Model file for the job. Use its own axes, mm. Face numbers are marked on the shaded views. Round coordinates to 2 decimals unless told otherwise and drop trailing zeros. Loops run counter-clockwise (first coordinate to the right, second up) from the corner with the lowest first, then second, coordinate; pieces in that order, holes last. Notation, with made-up numbers: (-11, -37.5) -> (17, -37.5) arc R24 cw to (17, -26.5) -> close; hole circle Ø4 at (-29.5, 39.25). An arc over 180 degrees is marked (long way). Use a Markdown table: item, result.
from build123d import *

# Parameters (mm, degrees)
SKETCH_1_W         = 40
SKETCH_1_H         = 40
EXTRUDE_1_DEPTH    = 4
HOLE_WIZARD_M101_D = 11
FILLET_1_R         = 3
HOLE_WIZARD_M61_D  = 6.6


with BuildPart() as part:
    # Эскиз1 → Бобышка-Вытянуть1 (new body)
    with BuildSketch(Plane(origin=(0, 0, 0), x_dir=(1, 0, 0), z_dir=(0, 1, 0))):
        Rectangle(SKETCH_1_W, SKETCH_1_H)
    extrude(amount=EXTRUDE_1_DEPTH)

    # Отверстие с зазором M101 (through all)
    with Locations(Plane(origin=(0, 4, 0), x_dir=(1, 0, 0), z_dir=(0, 1, 0))):
        with Locations((0, 0)):
            Hole(HOLE_WIZARD_M101_D / 2)

    # Скругление1
    fillet_1_edges = [part.edges().sort_by_distance(p)[0] for p in [
        (20, 2, 20),
        (-20, 2, 20),
        (-20, 2, -20),
        (20, 2, -20),
    ]]
    fillet(fillet_1_edges, radius=FILLET_1_R)

    # Отверстие с зазором M61 (through all)
    with Locations(Plane(origin=(0, 0, 0), x_dir=(-1, 0, 0), z_dir=(0, -1, 0))):
        with Locations((-14.5, 14.5), (0, 0), (14.5, 14.5), (-14.5, -14.5), (14.5, -14.5)):
            Hole(HOLE_WIZARD_M61_D / 2)


solid = part.part
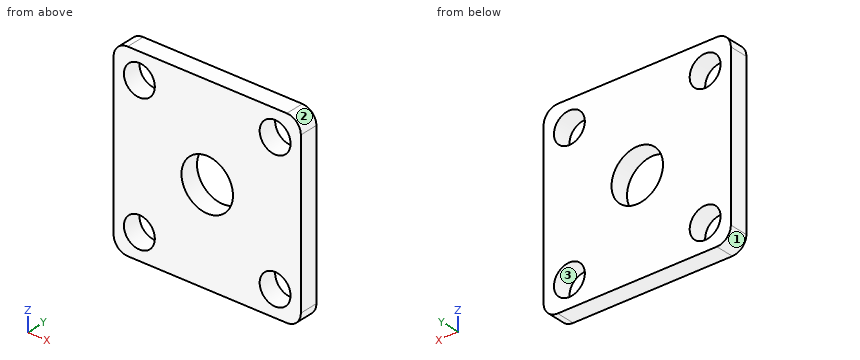
Q1. Band-saw the part on A-A, the plane x = -14.5. Give the cut face in (y, z), plus the area to 3 significant figures.
Results list:
| item | result |
|---|---|
| outline | (0, -20) -> (4, -20) -> (4, -17.8) -> (0, -17.8) -> close; (0, -11.2) -> (4, -11.2) -> (4, 11.2) -> (0, 11.2) -> close; (0, 17.8) -> (4, 17.8) -> (4, 20) -> (0, 20) -> close |
| area | 107 mm² |
Q2. Band-saw the part on B-B, the plane x = 0. Give the cut face in (y, z), plus the area to 3 significant figures.
Results list:
| item | result |
|---|---|
| outline | (0, -20) -> (4, -20) -> (4, -5.5) -> (0, -5.5) -> close; (0, 5.5) -> (4, 5.5) -> (4, 20) -> (0, 20) -> close |
| area | 116 mm² |
Q3. Band-saw the part on C-C, the plane z = 4. Give the cut face in (x, y), plus the area to 3 significant figures.
Results list:
| item | result |
|---|---|
| outline | (-20, 0) -> (-3.77, 0) -> (-3.77, 4) -> (-20, 4) -> close; (3.77, 0) -> (20, 0) -> (20, 4) -> (3.77, 4) -> close |
| area | 130 mm² |
Q4. Pull direction X, two halves, no side cores. Call the marked faces 1, 2 and 3: released by +X, released by -X, zero draft, split by the parting line, or undercut.
Results list:
| item | result |
|---|---|
| face 1 | released by -X |
| face 2 | released by +X |
| face 3 | undercut |
Q5. Drill centre lines: L1, parallel to X at y = 1.35, z = -14.5; L2, parallel to Z at x = 0, y = 3.05. Where is each one in solid material? Low to high. Write a range as from..to.
Results list:
| item | result |
|---|---|
| L1 | x = -20..-17.8, -11.2..11.2, 17.8..20 |
| L2 | z = -20..-5.5, 5.5..20 |
Q6. Band-saw the part on D-D, the plane y = 3.05. Give the cut face in (x, z), plus the area to 3 significant figures.
Results list:
| item | result |
|---|---|
| outline | (-20, -17) arc R3 ccw to (-17, -20) -> (17, -20) arc R3 ccw to (20, -17) -> (20, 17) arc R3 ccw to (17, 20) -> (-17, 20) arc R3 ccw to (-20, 17) -> close; hole circle Ø6.6 at (-14.5, -14.5); hole circle Ø6.6 at (-14.5, 14.5); hole circle Ø11 at (0, 0); hole circle Ø6.6 at (14.5, -14.5); hole circle Ø6.6 at (14.5, 14.5) |
| area | 1,360 mm² |
